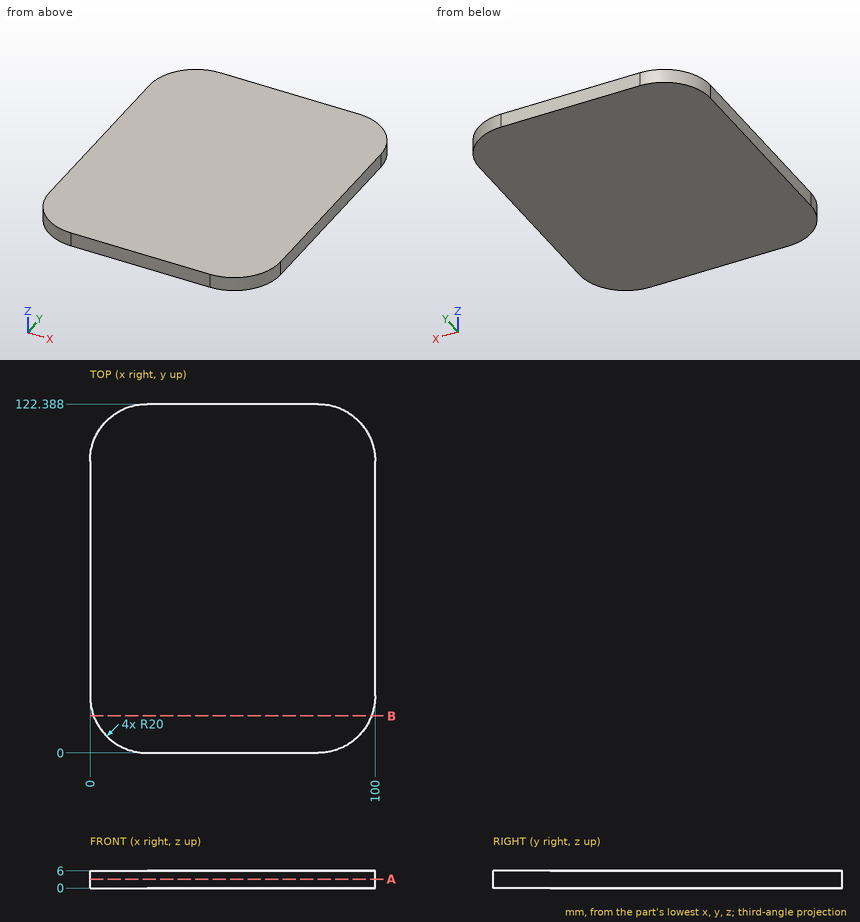
Geometry: see drawing. Coordinates: mm, zero at the bounding-box minimum. Round coordinates to 2 decimals unless told otherwise and drop trailing zeros. Loops run counter-clockwise (first coordinate to the right, second up) from the corner with the lowest first, then second, coordinate; pieces in that order, holes last. Notation, with made-up numbers: M -37.5,40 L 19.5,40 A26 cw 19.5,57 Z; hole C -6,9.5 d10. An arc over 180 degrees is marked long. Use a Markdown table: item, result. Add a question column.
1. Cut plane A-A, the plane z = 3.15. Output: boundary loops of the cut face in (x, y), and give its area (3 significant figures).
2. Cut plane B-B, the plane y = 13. Output: boundary loops of the cut face in (x, z) (3 decimals).
3. Ray query, line 1 along X through (y, z) = (103, 3); line 2 along Y through (x, z) = (7.5, 4); line 3 along Y through (x, z) = (18, 4.75). Return the intervals inside material, ascending. Write a range as [from, to].
Solution:
| question | item | result |
|---|---|---|
| 1 | outline | M 0,20 A20 ccw 20,0 L 80,0 A20 ccw 100,20 L 100,102.39 A20 ccw 80,122.39 L 20,122.39 A20 ccw 0,102.39 Z |
| 1 | area | 11,900 mm2 |
| 2 | outline | M 1.265,0 L 98.735,0 L 98.735,6 L 1.265,6 Z |
| 3 | line 1 | x = [0.01, 99.99] |
| 3 | line 2 | y = [4.39, 118] |
| 3 | line 3 | y = [0.1, 122.29] |
